```python
from build123d import *

# Parameters (mm, degrees)
SKETCH_2_W             = 100
SKETCH_2_H             = 43
EXTRUDE_1_DEPTH        = 8
SKETCH_3_R             = 5
CUT_EXTRUDE_1_DEPTH    = 8
HOLE_WIZARD_M6_1_D     = 5
HOLE_WIZARD_M6_1_DEPTH = 15
HOLE_WIZARD_M6_1_TIP   = 1.502151548
HOLE_WIZARD_M5_1_D     = 4.2
HOLE_WIZARD_M5_1_DEPTH = 12.4
HOLE_WIZARD_M5_1_TIP   = 1.2618073


with BuildPart() as part:
    # 草图2 → 凸台-拉伸1 (new body)
    with BuildSketch(Plane.XY):
        with Locations((50, 21.5)):
            Rectangle(SKETCH_2_W, SKETCH_2_H)
    extrude(amount=EXTRUDE_1_DEPTH)

    # 草图3 → 切除-拉伸1 (cut)
    with BuildSketch(Plane.XY.offset(8)):
        with Locations((50, 10)):
            Circle(SKETCH_3_R)
    extrude(amount=-CUT_EXTRUDE_1_DEPTH, mode=Mode.SUBTRACT)

    # M6 螺纹孔1
    with Locations(Plane.XY.offset(8)):
        with Locations((25, 10), (75, 10)):
            Hole(HOLE_WIZARD_M6_1_D / 2, depth=HOLE_WIZARD_M6_1_DEPTH)
            with Locations((0, 0, -(HOLE_WIZARD_M6_1_DEPTH + HOLE_WIZARD_M6_1_TIP / 2))):  # 118° drill point
                Cone(0, HOLE_WIZARD_M6_1_D / 2, HOLE_WIZARD_M6_1_TIP, mode=Mode.SUBTRACT)

    # M5 螺纹孔1
    with Locations(Plane(origin=(0, 43, 0), x_dir=(1, 0, 0), z_dir=(0, 1, 0))):
        with Locations((25, -4), (75, -4)):
            Hole(HOLE_WIZARD_M5_1_D / 2, depth=HOLE_WIZARD_M5_1_DEPTH)
            with Locations((0, 0, -(HOLE_WIZARD_M5_1_DEPTH + HOLE_WIZARD_M5_1_TIP / 2))):  # 118° drill point
                Cone(0, HOLE_WIZARD_M5_1_D / 2, HOLE_WIZARD_M5_1_TIP, mode=Mode.SUBTRACT)


solid = part.part
```
Source: CAD feature listing. Evaluate the final solid. Frame: model axes, mm. A direction names the side the tool comes from. Round coordinates to 2 decimals unless told otherwise and drop trailing zeros. Loops run counter-clockwise (first coordinate to the right, second up) from the corner with the lowest first, then second, coordinate; pieces in that order, holes last. Notation, with made-up numbers: M 62,-25.75 L 102,-25.75 A27 cw 102,11.25 Z; hole C 9,73 d9. An arc over 180 degrees is marked long. Use a Markdown table: item, result. Add a question column.
1. Section query B-B on y = 37. Return the cut outline in (x, z).
2. Mould query, pull axis Y, two halves, no side actions, for faces 3 (the conical face through (25.2, 29.56, 3.69)), 4 (the flat face through (49, 22, 8)), 5 (the cylindrical face through (77, 8.5, 3.9)). Classes: pulls with the +Y half, pulls with the -Y half, needs draft (parallel to the pull), parting line crosses it, or undercut.
3. Section query C-C on y = 8.5. Return the cut outline in (x, z).
4. Reachability of faces 1 (the flat face through (0, 21, 4)), 2 (the cylindrical face through (24.031, 36.713, 5.863)) from +Z, -Z, +X, -X, +Y, -Y: full face, straight path, thin tool, end or side. Return the list, or none.
5. Section query A-A on x = 50. Return the cut outline in (y, z), then the cut area to 3 significant figures.
6. Line query: line 1 (Y direction, x = 25, z = 6.5); line 2 (Y direction, x = 50, z = 2.25); line 3 (X direction, y = 36.5, z = 3). Output: solid intervals per line, ascending.
Reported:
| question | item | result |
|---|---|---|
| 1 | outline | M 0,0 L 100,0 L 100,8 L 0,8 Z; hole C 25,4 d4.2; hole C 75,4 d4.2 |
| 2 | face 3 | pulls with the +Y half |
| 2 | face 4 | needs draft |
| 2 | face 5 | undercut |
| 3 | outline | M 0,0 L 23,0 L 23,8 L 0,8 Z; M 27,0 L 45.23,0 L 45.23,8 L 27,8 Z; M 54.77,0 L 73,0 L 73,8 L 54.77,8 Z; M 77,0 L 100,0 L 100,8 L 77,8 Z |
| 4 | face 1 | +Z, -Z, -X, +Y, -Y |
| 4 | face 2 | +Y |
| 5 | outline | M 0,0 L 5,0 L 5,8 L 0,8 Z; M 15,0 L 43,0 L 43,8 L 15,8 Z |
| 5 | area | 264 mm² |
| 6 | line 1 | y = 0 to 7.5, 12.5 to 43 |
| 6 | line 2 | y = 0 to 5, 15 to 43 |
| 6 | line 3 | x = 0 to 23.15, 26.85 to 73.15, 76.85 to 100 |
